Design review of the part built by this model. Coordinates are the model's own, in mm. Face numbers are marked on the shaded views. A direction names the side the tool comes from. Give positions to 0.01 mm unless a question says otherwise; leave off trailing zeros. Loops run counter-clockwise (first coordinate to the right, second up) from the corner with the lowest first, then second, coordinate; pieces in that order, holes last. Notation, with made-up numbers: M -20.75,29.5 L -3.75,29.5 A13 cw -3.75,51.5 Z; hole C 23.5,19.5 d1. An arc over 180 degrees is marked long. Use one line per item in the form item = value. Start each with the question number.
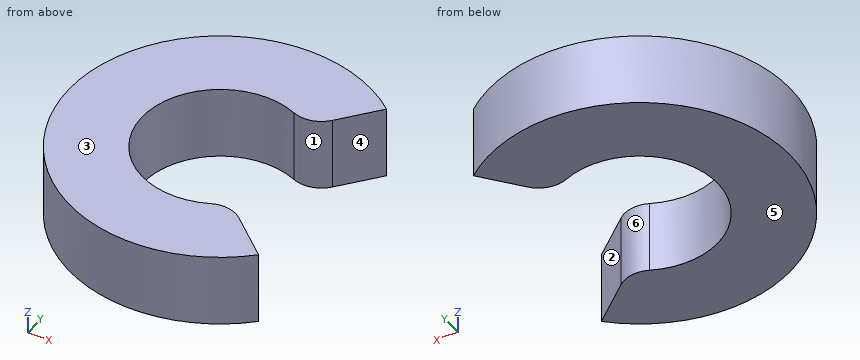
from build123d import *

# Parameters (mm, degrees)
F1_DEPTH = 12.7
F2_R     = 5.08


with BuildPart() as f1:
    # F0 (on Top) → F1 (new body)
    with BuildSketch(Plane.XY):
        with BuildLine():
            ThreePointArc((8.348858, -10.721823), (-13.589, 0), (8.348858, 10.721823))
            Line((8.348858, 10.721823), (16.617949, 20.370451))
            ThreePointArc((16.617949, 20.370451), (-26.270642, -0.982292), (18.092772, -19.072575))
            Line((18.092772, -19.072575), (8.348858, -10.721823))
        make_face()
    extrude(amount=F1_DEPTH)

    # F2
    f2_edges = [f1.edges().sort_by_distance(p)[0] for p in [
        (8.348858, 10.721823, 6.35),
        (8.348858, -10.721823, 6.35),
    ]]
    fillet(f2_edges, radius=F2_R)


solid = f1.part
Q1. For the marked faces 4, 5 and 6, list the 3-axis set-ups (+Z, -Z, +X, -X, +Y, -Y) from which the entire face can be reached by the end or side of a thin tool; tool diameter is ignored.
Q2. Take a section at C-C on z = 1. Give the boundary of the cut face in (x, y), plus the area to 3 significant figures.
Q3. The part is to be moulded in two halves that separate along X. For the marked faces 1, 2 and 3, say which applies: pulls with the +X half, pulls with the -X half, needs draft (parallel to the pull), parting line crosses it, or undercut.
Q4. Take a section at A-A on x = 0. Give the boundary of the cut face in (y, z).
Q5. Clearance check with flat-ended pins moving along their axes: pin 1 Ø2 at (y, z) = (-11, 6) entering from -X; pin 2 Ø6 at (x, z) = (-18, 3) entering from +Y; pin 3 Ø5 at (y, z) = (-16, 7.5) entering from +X. State where each tip first meets the part, or that it passes through.
Q6. Wall thickness on probe 1 along Y at (x, z) = (0, 6.5); probe 2 along X at (y, z) = (22.5, 9.5); probe 3 along X at (y, z) = (0, 7.25): over which ranges is each line inside the solid? List them lowest first.
Q7. Take a section at D-D on x = 7.5. Give the boundary of the cut face in (y, z).
Q8. Take a section at B-B on y = 0. Give the boundary of the cut face in (x, z), plus the area to 3 significant figures.
Response values:
q1.face_4 = +Z, -Z, +X
q1.face_5 = -Z, +X, -X, +Y, -Y
q1.face_6 = +Z, -Z
q2.outline = M 5.26,12.53 A5.08 ccw 11.08,13.91 L 16.62,20.37 A26.29 ccw long 18.09,-19.07 L 11.12,-13.1 A5.08 ccw 5.69,-12.34 A13.59 cw long Z
q2.area = 1,150 mm^2
q3.face_1 = undercut
q3.face_2 = pulls with the +X half
q3.face_3 = needs draft
q4.outline = M -26.29,0 L -13.59,0 L -13.59,12.7 L -26.29,12.7 Z; M 13.59,0 L 26.29,0 L 26.29,12.7 L 13.59,12.7 Z
q5.pin_1 = -24.31
q5.pin_2 = 21.59
q5.pin_3 = 17.42
q6.probe_1 = -26.29 to -13.59, 13.59 to 26.29
q6.probe_2 = -13.6 to 13.6
q6.probe_3 = -26.29 to -13.59
q7.outline = M -25.2,0 L -11.88,0 L -11.88,12.7 L -25.2,12.7 Z; M 12.14,0 L 25.2,0 L 25.2,12.7 L 12.14,12.7 Z
q8.outline = M -26.29,0 L -13.59,0 L -13.59,12.7 L -26.29,12.7 Z
q8.area = 161 mm^2
